Part print with two shaded views. Sizes in mm from the minimum x, y, z corner. A direction names the side the tool comes from. Give positions to 0.01 mm unless a question says otherwise; leave off trailing zeros. Write each loop counter-clockwise with the first axis right and the second up, starting at its lowest first coordinate (ties: lowest second). Pieces come first, ordered by that corner, then holes. Notation, with made-up numbers: (9.5, -29) -> (55.5, -29) arc R30 cw to (55.5, 5) -> close; hole circle Ø1 at (73.5, 73). An arc over 180 degrees is marked (long way). Answer as a JSON object with one key per item and string values.
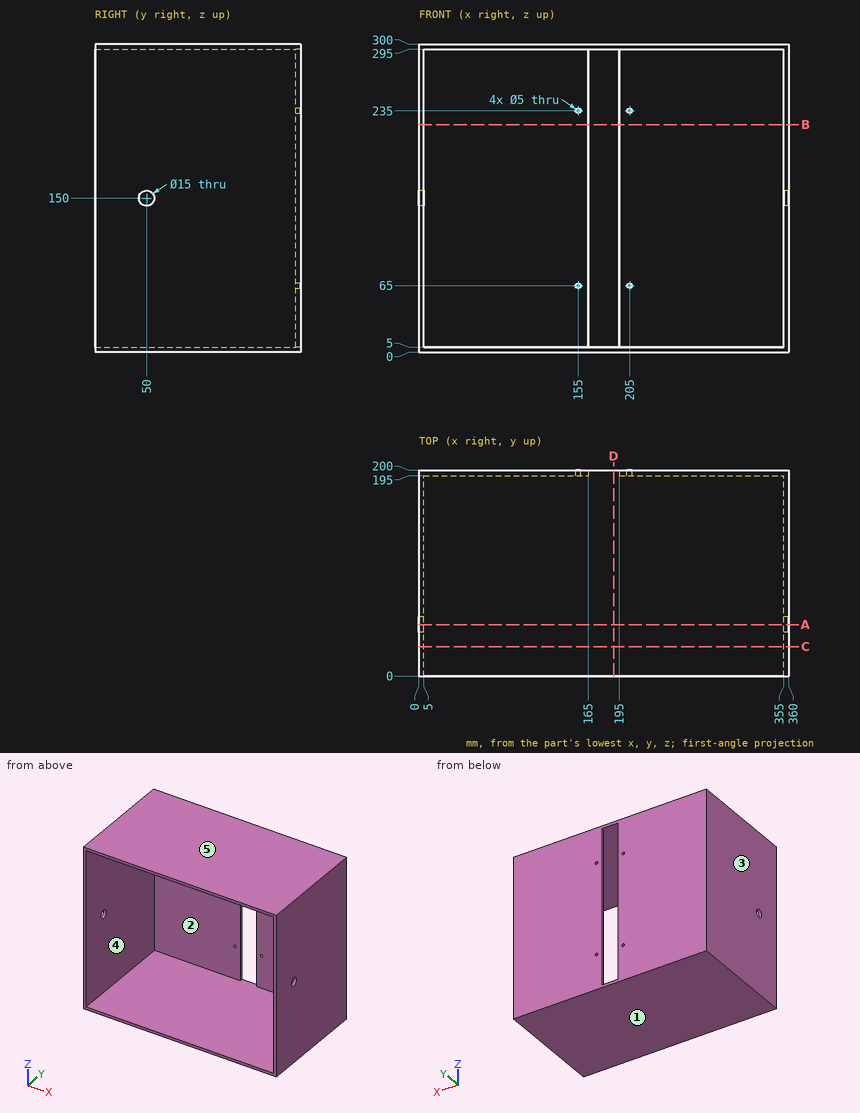
1) Pin check, flat tips, straight feed: pin 1 (10 mm diameter, centred on x = 205, z = 91.5, fed in from -Y); pin 2 (2.5 mm diameter, centred on y = 198.5, z = 172, fed in from -X); pin 3 (4.5 mm diameter, centred on x = 205, z = 65, fed in from +Y). Stop position of each tip, or through.
Model answer:
{"pin 1": "stops at y = 195", "pin 2": "stops at x = 0", "pin 3": "passes through"}
2) Mould opens along X. For the marked faces 3, 4 and 5 say: released by +X, released by -X, zero draft, split by the parting line, or undercut.
Model answer:
{"face 3": "released by -X", "face 4": "undercut", "face 5": "zero draft"}
3) Slice it at B-B (z = 221.5). List the corners of the cut face in (x, y), then the cut area to 3 significant figures.
Model answer:
{"outline": "(0, 0) -> (5, 0) -> (5, 195) -> (165, 195) -> (165, 200) -> (0, 200) -> close; (195, 195) -> (355, 195) -> (355, 0) -> (360, 0) -> (360, 200) -> (195, 200) -> close", "area": "3,600 mm2"}
4) Slice it at D-D (x = 189.5). List the corners of the cut face in (y, z), then the cut area to 3 significant figures.
Model answer:
{"outline": "(0, 0) -> (200, 0) -> (200, 5) -> (0, 5) -> close; (0, 295) -> (200, 295) -> (200, 300) -> (0, 300) -> close", "area": "2,000 mm2"}
5) Wall check: probe 1 along X at (y, z) = (197.25, 65); probe 2 along Z at (x, y) = (205, 198); probe 3 along Z at (x, y) = (256, 140). Give the ranges that are in metal, low to high.
Model answer:
{"probe 1": "x = 0 to 152.5, 157.5 to 165, 195 to 202.5, 207.5 to 360", "probe 2": "z = 0 to 62.5, 67.5 to 232.5, 237.5 to 300", "probe 3": "z = 0 to 5, 295 to 300"}
6) Slice it at A-A (y = 50). List the corners of the cut face in (x, z).
Model answer:
{"outline": "(0, 0) -> (360, 0) -> (360, 142.5) -> (355, 142.5) -> (355, 5) -> (5, 5) -> (5, 142.5) -> (0, 142.5) -> close; (0, 157.5) -> (5, 157.5) -> (5, 295) -> (355, 295) -> (355, 157.5) -> (360, 157.5) -> (360, 300) -> (0, 300) -> close"}
7) Slice it at C-C (y = 28.5). List the corners of the cut face in (x, z).
Model answer:
{"outline": "(0, 0) -> (360, 0) -> (360, 300) -> (0, 300) -> close; hole (5, 5) -> (355, 5) -> (355, 295) -> (5, 295) -> close"}
8) 3-axis set-ups, long thin cutter, end or side, ignore diameter. For the marked faces 1 and 2: which of +Z, -Z, +X, -X, +Y, -Y reach the whole face in a straight line?
Model answer:
{"face 1": "-Z, +X, -X, +Y, -Y", "face 2": "-Y"}
